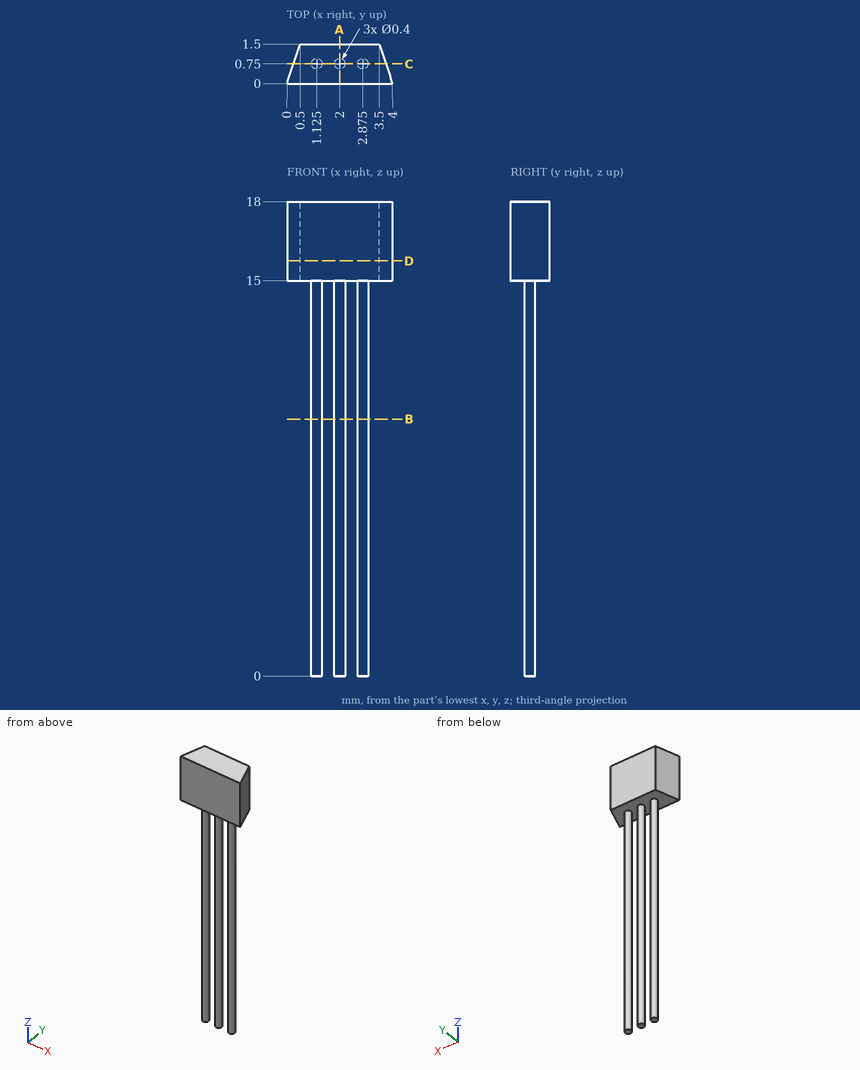
Job drawing, mm, ordinate dimensions from the low corner. One solid piece. Coordinates: 2 decimals unless noted, no trailing zeros. Order: outer loops, then holes, each group sorted by start corner. A loop starts at its lowest first (then second) coordinate and runs counter-clockwise, first axis right, second up. Notation, with made-up numbers: (-35, -15.5) - (-1, -15.5) arc R20 cw to (-1, 13.5) - close; hole circle Ø5 at (53, 37.5). An arc over 180 degrees is marked (long way). Write each question's results on one line, items separated by ' | '. Start each with the question number.
Item 1: Wall check: probe 1 along Z at (x, y) = (1.05, 1.2); probe 2 along Y at (x, z) = (1.1, 5); probe 3 along X at (y, z) = (0.8, 17). Give the ranges that are in metal, low to high. Write a range as [from, to].
Item 2: Band-saw the part on D-D on z = 15.75. Write the cut outline in (x, y).
Item 3: Band-saw the part on B-B on z = 9.75. Write the cut outline in (x, y) (3 decimals), and give its area (3 significant figures).
Item 4: Band-saw the part on A-A on x = 2. Write the cut outline in (y, z), and give its area (3 significant figures).
Item 5: Band-saw the part on C-C on y = 0.75. Write the cut outline in (x, z) (3 decimals).
Numbers:
1) probe 1: [15, 18] | probe 2: [0.55, 0.95] | probe 3: [0.27, 3.73]
2) outline: (0, 0) - (4, 0) - (3.5, 1.5) - (0.5, 1.5) - close
3) outline: circle Ø0.4 at (1.125, 0.75); circle Ø0.4 at (2, 0.75); circle Ø0.4 at (2.875, 0.75) | area: 0.377 mm^2
4) outline: (0, 15) - (0.55, 15) - (0.55, 0) - (0.95, 0) - (0.95, 15) - (1.5, 15) - (1.5, 18) - (0, 18) - close | area: 10.5 mm^2
5) outline: (0.25, 15) - (0.925, 15) - (0.925, 0) - (1.325, 0) - (1.325, 15) - (1.8, 15) - (1.8, 0) - (2.2, 0) - (2.2, 15) - (2.675, 15) - (2.675, 0) - (3.075, 0) - (3.075, 15) - (3.75, 15) - (3.75, 18) - (0.25, 18) - close
